Geometry: final body of the model. Coordinates: model frame, mm. Face numbers are marked on the shaded views. A direction names the side the tool comes from. Round coordinates to 2 decimals unless told otherwise and drop trailing zeros. Write each loop counter-clockwise with the first axis right and the second up, starting at its lowest first coordinate (ties: lowest second). Pieces come first, ordered by that corner, then holes. Notation, with made-up numbers: M 45,-30 L 82,-30 A27 cw 82,-2 Z; hole C 35,68 d8. An arc over 180 degrees is marked long. Use one line per item in the form item = value. Start each with the question number.
Item 1: Section query A-A (x = 58). Return loops of the section in (y, z), and give its area (3 significant figures).
Item 2: Ray query, probe 1 along X at (y, z) = (8.5, 0); probe 2 along X at (y, z) = (1.95, -43.5); probe 3 along X at (y, z) = (2.05, -43.5). Return the intervals inside material, ascending.
Item 3: Pin query (flat end, axial travel): pin 1 Ø4 at (x, z) = (97, -43.5) entering from -Y; pin 2 Ø2 at (x, z) = (66.5, 15) entering from +Y; pin 3 Ø3 at (x, z) = (-59.5, 19) entering from +Y; pin 4 Ø4 at (x, z) = (54, -36.5) entering from -Y. Return the tip coordinate at first contact, or that it passes through.
Item 4: Section query B-B (z = 2). Return loops of the section in (x, y).
Item 5: Reachability of the marked faces 1, 2, 3, 4 and 5 from +Z, -Z, +X, -X, +Y, -Y: full face, straight path, thin tool, end or side. Return the list, or none.
Item 6: Section query C-C (x = 33.5). Return loops of the section in (y, z).
Item 7: Section query D-D (z = 24.5). Return loops of the section in (x, y).
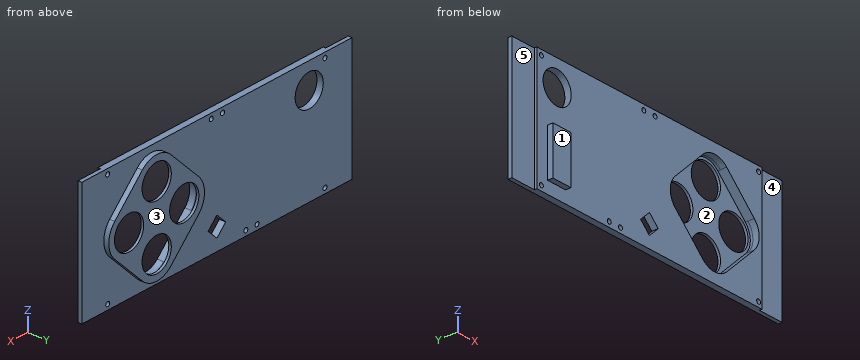
from build123d import *

# Parameters (mm, degrees)
SKETCH1_W           = 200
SKETCH1_H           = 95
SKETCH1_R           = 1.75
BOSS_EXTRUDE1_DEPTH = 5
SKETCH2_R           = 15
SKETCH2_R_2         = 12.5
CUT_EXTRUDE1_DEPTH  = 5
SKETCH4_W           = 16
SKETCH4_H           = 37
BOSS_EXTRUDE2_DEPTH = 4.2
SKETCH6_W           = 20
SKETCH6_H           = 95
BOSS_EXTRUDE3_DEPTH = 3
BOSS_EXTRUDE4_START = 4
BOSS_EXTRUDE4_DEPTH = 4
SKETCH9_R           = 13
BOSS_EXTRUDE5_DEPTH = 2
CUT_EXTRUDE2_DEPTH  = 5
SKETCH11_R          = 1.75
CUT_EXTRUDE3_DEPTH  = 10


with BuildPart() as part:
    # Sketch1 → Boss-Extrude1 (new body)
    with BuildSketch(Plane(origin=(0, 0, 0), x_dir=(1, 0, 0), z_dir=(0, 1, 0))):
        Rectangle(SKETCH1_W, SKETCH1_H)
        with Locations(Location((-96, 43.5, 0), (0, 0, 270))):
            Circle(SKETCH1_R, mode=Mode.SUBTRACT)
        with Locations(Location((-96, -43.5, 0), (0, 0, 270))):
            Circle(SKETCH1_R, mode=Mode.SUBTRACT)
        with Locations(Location((97, 43.5, 0), (0, 0, 270))):
            Circle(SKETCH1_R, mode=Mode.SUBTRACT)
        with Locations(Location((97, -43.5, 0), (0, 0, 270))):
            Circle(SKETCH1_R, mode=Mode.SUBTRACT)
    extrude(amount=BOSS_EXTRUDE1_DEPTH)

    # Sketch2 → Cut-Extrude1 (cut)
    with BuildSketch(Plane(origin=(0, 5, 0), x_dir=(1, 0, 0), z_dir=(0, 1, 0))):
        with Locations((33.5, 0)):
            Circle(SKETCH2_R)
        with BuildLine():
            ThreePointArc((48.5, 0), (39.240251485, -13.858192988), (22.893398282, -10.606601718))
            Line((22.893398282, -10.606601718), (47.393398282, -35.106601718))
            ThreePointArc((47.393398282, -35.106601718), (52.259748515, -10.641807012), (73, -24.5))
            ThreePointArc((73, -24.5), (71.858192988, -30.240251485), (68.606601718, -35.106601718))
            Line((68.606601718, -35.106601718), (93.106601718, -10.606601718))
            ThreePointArc((93.106601718, -10.606601718), (67.5, 0), (93.106601718, 10.606601718))
            Line((93.106601718, 10.606601718), (68.606601718, 35.106601718))
            ThreePointArc((68.606601718, 35.106601718), (71.858192988, 30.240251485), (73, 24.5))
            ThreePointArc((73, 24.5), (52.259748515, 10.641807012), (47.393398282, 35.106601718))
            Line((47.393398282, 35.106601718), (22.893398282, 10.606601718))
            ThreePointArc((22.893398282, 10.606601718), (39.240251485, 13.858192988), (48.5, 0))
        make_face()
        with Locations((58, -24.5)):
            Circle(SKETCH2_R)
        with Locations((82.5, 0)):
            Circle(SKETCH2_R)
        with Locations((58, 24.5)):
            Circle(SKETCH2_R)
        with Locations(Location((-82, -27.5, 0), (0, 0, 270))):
            Circle(SKETCH2_R_2)
    extrude(amount=-CUT_EXTRUDE1_DEPTH, mode=Mode.SUBTRACT)

    # Sketch4 → Boss-Extrude2 (add)
    with BuildSketch(Plane.XZ):
        with Locations((-82.5, -19.5)):
            Rectangle(SKETCH4_W, SKETCH4_H)
    extrude(amount=BOSS_EXTRUDE2_DEPTH)

    # Sketch6 → Boss-Extrude3 (add)
    with BuildSketch(Plane(origin=(0, 5, 0), x_dir=(1, 0, 0), z_dir=(0, 1, 0))):
        with Locations((-110, 0)):
            Rectangle(SKETCH6_W, SKETCH6_H)
        with Locations((110, 0)):
            Rectangle(SKETCH6_W, SKETCH6_H)
    extrude(amount=-BOSS_EXTRUDE3_DEPTH)

    # Sketch8 → Boss-Extrude4 (add)
    with BuildSketch(Plane(origin=(0, 5, 0), x_dir=(1, 0, 0), z_dir=(0, 1, 0)).offset(BOSS_EXTRUDE4_START)):
        with BuildLine():
            Line((70.727922061, -37.227922061), (95.227922061, -12.727922061))
            ThreePointArc((95.227922061, -12.727922061), (100.5, 0), (95.227922061, 12.727922061))
            Line((95.227922061, 12.727922061), (70.727922061, 37.227922061))
            ThreePointArc((70.727922061, 37.227922061), (58, 42.5), (45.272077939, 37.227922061))
            Line((45.272077939, 37.227922061), (20.772077939, 12.727922061))
            ThreePointArc((20.772077939, 12.727922061), (15.5, 0), (20.772077939, -12.727922061))
            Line((20.772077939, -12.727922061), (45.272077939, -37.227922061))
            ThreePointArc((45.272077939, -37.227922061), (58, -42.5), (70.727922061, -37.227922061))
        make_face()
        with BuildLine():
            Line((22.893398282, -10.606601718), (47.393398282, -35.106601718))
            ThreePointArc((47.393398282, -35.106601718), (58, -39.5), (68.606601718, -35.106601718))
            Line((68.606601718, -35.106601718), (93.106601718, -10.606601718))
            ThreePointArc((93.106601718, -10.606601718), (97.5, 0), (93.106601718, 10.606601718))
            Line((93.106601718, 10.606601718), (68.606601718, 35.106601718))
            ThreePointArc((68.606601718, 35.106601718), (58, 39.5), (47.393398282, 35.106601718))
            Line((47.393398282, 35.106601718), (22.893398282, 10.606601718))
            ThreePointArc((22.893398282, 10.606601718), (18.5, 0), (22.893398282, -10.606601718))
        make_face(mode=Mode.SUBTRACT)
    extrude(amount=-BOSS_EXTRUDE4_DEPTH)

    # Sketch9 → Boss-Extrude5 (add)
    with BuildSketch(Plane(origin=(0, 9, 0), x_dir=(1, 0, 0), z_dir=(0, 1, 0))):
        with BuildLine():
            Line((22.893398282, -10.606601718), (47.393398282, -35.106601718))
            ThreePointArc((47.393398282, -35.106601718), (58, -39.5), (68.606601718, -35.106601718))
            Line((68.606601718, -35.106601718), (93.106601718, -10.606601718))
            ThreePointArc((93.106601718, -10.606601718), (97.5, 0), (93.106601718, 10.606601718))
            Line((93.106601718, 10.606601718), (68.606601718, 35.106601718))
            ThreePointArc((68.606601718, 35.106601718), (58, 39.5), (47.393398282, 35.106601718))
            Line((47.393398282, 35.106601718), (22.893398282, 10.606601718))
            ThreePointArc((22.893398282, 10.606601718), (18.5, 0), (22.893398282, -10.606601718))
        make_face()
        with Locations(Location((58, 24.5, 0), (0, 0, 270))):
            Circle(SKETCH9_R, mode=Mode.SUBTRACT)
        with Locations(Location((82.5, 0, 0), (0, 0, 270))):
            Circle(SKETCH9_R, mode=Mode.SUBTRACT)
        with Locations(Location((58, -24.5, 0), (0, 0, 270))):
            Circle(SKETCH9_R, mode=Mode.SUBTRACT)
        with Locations(Location((33.5, 0, 0), (0, 0, 270))):
            Circle(SKETCH9_R, mode=Mode.SUBTRACT)
    extrude(amount=-BOSS_EXTRUDE5_DEPTH)

    # Sketch10 → Cut-Extrude2 (cut)
    with BuildSketch(Plane(origin=(0, 5, 0), x_dir=(1, 0, 0), z_dir=(0, 1, 0))):
        Polygon((0, 38.5), (-7.778174593, 30.721825407), (0, 22.943650814), (7.778174593, 30.721825407), align=None)
    extrude(amount=-CUT_EXTRUDE2_DEPTH, mode=Mode.SUBTRACT)

    # Sketch11 → Cut-Extrude3 (cut)
    with BuildSketch(Plane(origin=(0, 5, 0), x_dir=(1, 0, 0), z_dir=(0, 1, 0))):
        with Locations(Location((-35.721825407, 43.5, 0), (0, 0, 270))):
            Circle(SKETCH11_R)
        with Locations(Location((-25.721825407, 43.5, 0), (0, 0, 270))):
            Circle(SKETCH11_R)
        with Locations(Location((5, -43.5, 0), (0, 0, 270))):
            Circle(SKETCH11_R)
        with Locations(Location((-5, -43.5, 0), (0, 0, 270))):
            Circle(SKETCH11_R)
    extrude(amount=-CUT_EXTRUDE3_DEPTH, mode=Mode.SUBTRACT)


solid = part.part
Working result:
q1.outline = M 0,-47.5 L 5,-47.5 L 5,-42.5 L 9,-42.5 L 9,-37.5 L 7,-37.5 L 7,-39.5 L 0,-39.5 Z; M 0,39.5 L 7,39.5 L 7,37.5 L 9,37.5 L 9,42.5 L 5,42.5 L 5,47.5 L 0,47.5 Z; M 7,-11.5 L 9,-11.5 L 9,11.5 L 7,11.5 Z
q1.area = 158 mm²
q2.probe_1 = 15.5 to 20.5, 46.5 to 69.5, 95.5 to 100.5
q2.probe_2 = -100 to -97.75, -94.25 to -37.47, -33.97 to -27.47, -23.97 to 95.25, 98.75 to 100
q2.probe_3 = -120 to -97.75, -94.25 to -37.47, -33.97 to -27.47, -23.97 to 95.25, 98.75 to 120
q3.pin_1 = 0
q3.pin_2 = 9
q3.pin_3 = 5
q3.pin_4 = 7
q4.outline = M -120,2 L -100,2 L -100,0 L 18.63,0 L 18.63,7 L 20.65,7 L 20.65,9 L 15.61,9 L 15.61,5 L -120,5 Z; M 46.35,7 L 69.65,7 L 69.65,9 L 46.35,9 Z; M 95.35,7 L 97.37,7 L 97.37,0 L 100,0 L 100,2 L 120,2 L 120,5 L 100.39,5 L 100.39,9 L 95.35,9 Z
q5.face_1 = +Z, -Z, +X, -X, -Y
q5.face_2 = -Y
q5.face_3 = +Z, -Z, +X, -X, +Y
q5.face_4 = +Z, -Z, +X, -Y
q5.face_5 = +Z, -Z, -X, -Y
q6.outline = M 0,-47.5 L 5,-47.5 L 5,-25.46 L 9,-25.46 L 9,-13 L 7,-13 L 7,-21.21 L 0,-21.21 Z; M 0,21.21 L 7,21.21 L 7,13 L 9,13 L 9,25.46 L 5,25.46 L 5,47.5 L 0,47.5 Z
q7.outline = M -120,2 L -100,2 L -100,0 L -94.13,0 L -94.13,5 L -120,5 Z; M -69.87,0 L 36.79,0 L 36.79,7 L 45,7 L 45,9 L 32.54,9 L 32.54,5 L -69.87,5 Z; M 71,7 L 79.21,7 L 79.21,0 L 100,0 L 100,2 L 120,2 L 120,5 L 83.46,5 L 83.46,9 L 71,9 Z
